from build123d import *

# Parameters (mm, degrees)
BOSS_EXTRUDE1_DEPTH = 12.7
SKETCH2_R           = 2.24536
SKETCH2_W           = 12.7
SKETCH2_H           = 12.7
CUT_EXTRUDE1_DEPTH  = 57.115223473


with BuildPart() as part:
    # Sketch1 → Boss-Extrude1 (new body)
    with BuildSketch(Plane.XY):
        Polygon((-32.163183971, -6.040112022), (-32.163183971, -30.603981495), (31.336816029, -30.603981495), (31.336816029, -6.040112022), (44.036816029, -6.040112022), (44.036816029, 19.359887978), (31.336816029, 19.359887978), (31.336816029, 31.223757452), (-32.163183971, 31.223757452), (-32.163183971, 19.359887978), (-44.863183971, 19.359887978), (-44.863183971, -6.040112022), align=None)
    extrude(amount=BOSS_EXTRUDE1_DEPTH)

    # Sketch2 → Cut-Extrude1 (cut, through all)
    with BuildSketch(Plane.XY.offset(12.7)):
        with Locations((-5.273629901, -9.966481495)):
            Circle(SKETCH2_R)
        with Locations((-5.273629901, -19.491481495)):
            Circle(SKETCH2_R)
        with Locations((4.251370099, -19.491481495)):
            Circle(SKETCH2_R)
        with Locations((4.251370099, -9.966481495)):
            Circle(SKETCH2_R)
        with Locations((-0.511129901, -14.728981495)):
            Rectangle(SKETCH2_W, SKETCH2_H)
    extrude(amount=-CUT_EXTRUDE1_DEPTH, mode=Mode.SUBTRACT)


solid = part.part
Geometry check sheet. Reference: the model listing, model coordinates, mm. A direction names the side the tool comes from. Round coordinates to 2 decimals unless told otherwise and drop trailing zeros. Write each loop counter-clockwise with the first axis right and the second up, starting at its lowest first coordinate (ties: lowest second). Pieces come first, ordered by that corner, then holes. Notation, with made-up numbers: (11, 41) -> (56, 41) arc R8 cw to (56, 50) -> close; hole circle Ø1 at (70.25, 30.5). An arc over 180 degrees is marked (long way). One line per item, written item: value. Start each with the question number.
(1) Cross-section at A-A, the plane z = 2. Record the cut outline in (x, y), and give its area (3 significant figures).
(2) Draft check along X on faces 4 (the flat face through (-44.863, 7, 6)), 5 (the flat face through (38, 19.36, 6)), 6 (the cylindrical face through (5.804, -21.114, 6.439)). Enter one of: +X half, -X half, draft (parallel to the pull), parting line (faces both ways), or undercut.
(3) Go/stop test with flat-tipped pins: pin 1 Ø4 at (x, z) = (-35.5, 9) entering from -Y; pin 2 Ø4 at (y, z) = (-22.5, 4) entering from -X; pin 3 Ø6.5 at (x, z) = (36.5, 5.5) entering from +Y. Record where each tip stops, or that it passes through.
(4) Scan lines: line 1 (X direction, y = -17, z = 7.5); line 2 (Y direction, x = 39, z = 0.5); line 3 (Y direction, x = -6.5, z = 10.75). Record each from-to range of solid material in increasing order. Write a range as [from, to].
(5) Access from +Z, -Z, +X, -X, +Y, -Y to the whole of each face (thin tool, end or side, straight path). Record for faces 1 (the flat face through (-39, -6.04, 6)), 2 (the flat face through (31.337, -18, 6)), 3 (the flat face through (-6.861, -15, 6)).
(6) Cross-section at C-C, the plane x = -35.5. Record the cut outline in (y, z), and give its area (3 significant figures).
(7) Cross-section at D-D, the plane y = -19. Record the cut outline in (x, z), and give its area (3 significant figures).
(8) Cross-section at B-B, the plane y = -9.5. Record the cut outline in (x, z), and give its area (3 significant figures).
Answer:
1. outline: (-44.86, -6.04) -> (-32.16, -6.04) -> (-32.16, -30.6) -> (31.34, -30.6) -> (31.34, -6.04) -> (44.04, -6.04) -> (44.04, 19.36) -> (31.34, 19.36) -> (31.34, 31.22) -> (-32.16, 31.22) -> (-32.16, 19.36) -> (-44.86, 19.36) -> close; hole (-6.86, -17.9) arc R2.25 ccw to (-3.69, -21.08) -> (2.66, -21.08) arc R2.25 ccw to (5.84, -17.9) -> (5.84, -11.55) arc R2.25 ccw to (2.66, -8.38) -> (-3.69, -8.38) arc R2.25 ccw to (-6.86, -11.55) -> close
1. area: 4,400 mm²
2. face 4: -X half
2. face 5: draft
2. face 6: undercut
3. pin 1: y = -6.04
3. pin 2: x = -32.16
3. pin 3: y = 19.36
4. line 1: [-32.16, -6.86], [5.84, 31.34]
4. line 2: [-6.04, 19.36]
4. line 3: [-30.6, -21.37], [-8.09, 31.22]
5. face 1: +Z, -Z, -X, -Y
5. face 2: +Z, -Z, +X, -Y
5. face 3: +Z, -Z
6. outline: (-6.04, 0) -> (19.36, 0) -> (19.36, 12.7) -> (-6.04, 12.7) -> close
6. area: 323 mm²
7. outline: (-32.16, 0) -> (-7.46, 0) -> (-7.46, 12.7) -> (-32.16, 12.7) -> close; (6.44, 0) -> (31.34, 0) -> (31.34, 12.7) -> (6.44, 12.7) -> close
7. area: 630 mm²
8. outline: (-32.16, 0) -> (-7.47, 0) -> (-7.47, 12.7) -> (-32.16, 12.7) -> close; (6.45, 0) -> (31.34, 0) -> (31.34, 12.7) -> (6.45, 12.7) -> close
8. area: 630 mm²
